```python
from build123d import *

# Parameters (mm, degrees)
F1_DEPTH = 2


with BuildPart() as f1:
    # F0 (on Front) → F1 (new body)
    with BuildSketch(Plane.XZ):
        with BuildLine():
            Line((-2.5, 24.7390419245), (-2.5, 3.1224989992))
            ThreePointArc((-2.5, 3.1224989992), (-3.7742546282, -1.3247648854), (0, -4))
            ThreePointArc((0, -4), (3.7742546282, -1.3247648854), (2.5, 3.1224989992))
            Line((2.5, 3.1224989992), (2.5, 24.7390419245))
            add(Edge.make_bspline(
                [(0, 35), (2.6780768056, 32.0475395766), (7.0401936793, 27.2384997362), (3.7645832593, 25.4352175715), (2.5, 24.7390419245)],
                knots=[0, 0, 0, 0, 0.6139396742, 1, 1, 1, 1], degree=3))
            add(Edge.make_bspline(
                [(0, 35), (-2.6780768056, 32.0475395766), (-7.0401936793, 27.2384997362), (-3.7645832593, 25.4352175715), (-2.5, 24.7390419245)],
                knots=[0, 0, 0, 0, 0.6139396742, 1, 1, 1, 1], degree=3))
        make_face()
        with BuildLine():
            ThreePointArc((0, -1.5191429047), (-1.5191429047, 0), (0, 1.5191429047))
            ThreePointArc((0, 1.5191429047), (1.5191429047, 0), (0, -1.5191429047))
        make_face(mode=Mode.SUBTRACT)
        with BuildLine():
            add(Edge.make_bspline(
                [(0, 31.1435163021), (-1.2354901485, 29.1288048963), (-3.2717680855, 25.8082507742), (-0.9234860023, 26.5364242479), (0, 26.8227867782)],
                knots=[0, 0, 0, 0, 0.6067394335, 1, 1, 1, 1], degree=3))
            add(Edge.make_bspline(
                [(0, 31.1435163021), (1.2354901485, 29.1288048963), (3.2717680855, 25.8082507742), (0.9234860023, 26.5364242479), (0, 26.8227867782)],
                knots=[0, 0, 0, 0, 0.6067394335, 1, 1, 1, 1], degree=3))
        make_face(mode=Mode.SUBTRACT)
    extrude(amount=F1_DEPTH)


solid = f1.part
```
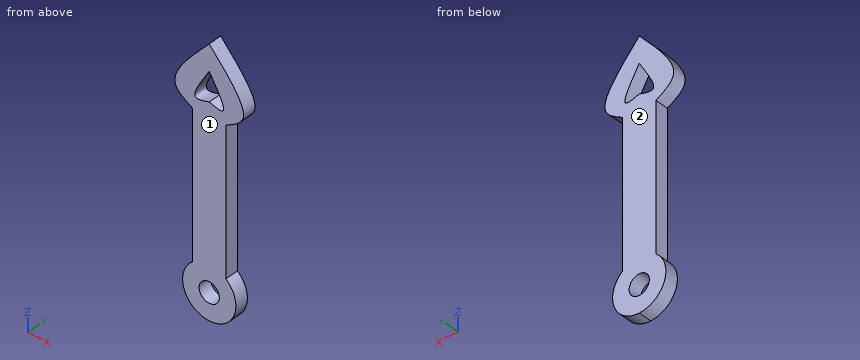
Read the model definition and answer for the solid it produces. Units are mm, in the model's axes. Face numbers are marked on the shaded views. Give positions to 0.01 mm unless a question says otherwise; leave off trailing zeros. Order: outer loops, then holes, each group sorted by start corner. A loop starts at its lowest first (then second) coordinate and runs counter-clockwise, first axis right, second up.
(1) Straight lines are drawn through the part: L1, parallel to X at y = -1, z = 0; L2, parallel to Z at x = -3.25, y = -0.7; L3, parallel to Z at x = -3.5, y = -0.7. For each, find the intervals that lie inside material, in ascending order.
(2) Given pin 1 (1 mm diameter, centred on y = -1, z = 9.5, fed in from -X); pin 2 (1.8 mm diameter, centred on x = 0, z = 0, fed in from -Y), each flat-ended and moving along its own axis, determine where each tip first touches the part or whether it passes through.
(3) Find section C-C (x = -1). Give the number of separate pieces and of enclosed holes in the cut face, plus the area to 3 significant figures.
(4) Find section A-A (z = 0). Give the vertices of the cut face in (x, y).
(5) For a pull along Y with two mould halves and no side action, classify the marked faces 1 and 2 as released by +Y, released by -Y, zero draft, split by the parting line, or undercut.
(6) Find section B-B (z = 14). Give the vertices of the cut face in (x, y), plus the area to 3 significant figures.
Result sheet:
1. L1: x = -4 to -1.52, 1.52 to 4
1. L2: z = -2.33 to 2.33, 25.16 to 31.25
1. L3: z = -1.94 to 1.94, 25.31 to 30.92
2. pin 1: stops at x = -2.5
2. pin 2: passes through
3. separate pieces: 3
3. enclosed holes: 0
3. area: 65.1 mm2
4. outline: (-4, -2) - (-1.52, -2) - (-1.52, 0) - (-4, 0) - close; (1.52, -2) - (4, -2) - (4, 0) - (1.52, 0) - close
5. face 1: released by -Y
5. face 2: released by +Y
6. outline: (-2.5, -2) - (2.5, -2) - (2.5, 0) - (-2.5, 0) - close
6. area: 10.0 mm2
